Read the model definition and answer for the solid it produces. Units are mm, in the model's axes. Give positions to 0.01 mm unless a question says otherwise; leave off trailing zeros. Loops run counter-clockwise (first coordinate to the right, second up) from the corner with the lowest first, then second, coordinate; pieces in that order, holes last. Notation, with made-up numbers: (74, -12) - (128, -12) arc R19 ccw to (128, 0) - close; hole circle Ø7 at (-33, 36.25). An arc over 180 degrees is marked (long way). Use a Markdown table: item, result. Add a question column.
Item 1: A cutting plane is placed at D-D (z = 2.25). Give the number of separate pieces and of enclosed holes in the cut face, plus the area to 3 significant figures.
Item 2: A cutting plane is placed at A-A (x = 0). Determine the outline of the cut face in (y, z).
Item 3: Each of these flat-tipped pins is pushed along its axis until it touches: P1, Ø1.5, axis at x = 10, z = 2, coming from the -Y side; P2, Ø3, axis at y = -18, z = 1.5, coming from the +X side; P3, Ø2, axis at x = 0.5, z = 3.5, coming from the +Y side. Where does it stop, or does it pass through?
Item 4: Consider probe 1 along Y at (x, z) = (0, 3.2); probe 2 along X at (y, z) = (11.5, 1.15); probe 3 along X at (y, z) = (13, 1.2). Determine where each line is inside the solid, lowest interval first. Write a range as [from, to].
Item 5: A cutting plane is placed at C-C (x = 15). Determine the outline of the cut face in (y, z).
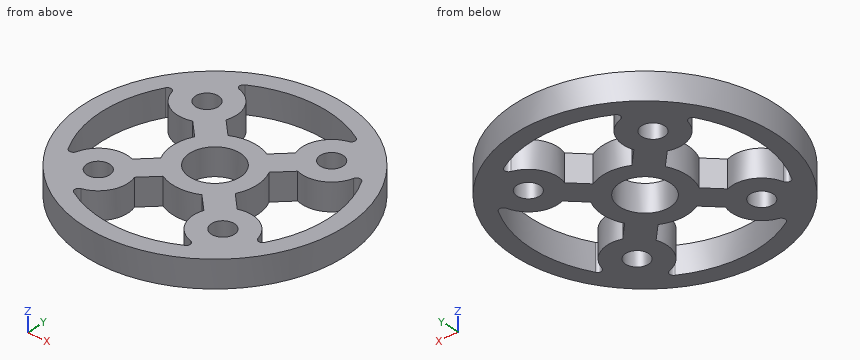
from build123d import *

# Parameters (mm, degrees)
F0_R            = 24.51608
F0_R_2          = 2.15265
F0_R_3          = 4.7625
F1_DEPTH        = 5.08
F3_DEPTH        = 5.08
F3_COPIES_COUNT = 4
F4_R            = 0.762


# Not quite as in the source:
# - a pattern or mirror of a feature is missing from the dataset's text; its kind, count and spacing are read off the source's solid


with BuildPart() as f1:
    # F0 (on Top) → F1 (new body)
    with BuildSketch(Plane.XY):
        Circle(F0_R)
        with Locations((-11.7865906, -11.7865906)):
            Circle(F0_R_2, mode=Mode.SUBTRACT)
        with Locations((11.7865906, -11.7865906)):
            Circle(F0_R_2, mode=Mode.SUBTRACT)
        with Locations((-11.7865906, 11.7865906)):
            Circle(F0_R_2, mode=Mode.SUBTRACT)
        Circle(F0_R_3, mode=Mode.SUBTRACT)
        with Locations((11.7865906, 11.7865906)):
            Circle(F0_R_2, mode=Mode.SUBTRACT)
    extrude(amount=F1_DEPTH)

    # F2 (on face) → F3 (cut, through all)
    with BuildSketch(Plane.XY.offset(5.08)):
        with BuildLine():
            ThreePointArc((-12.5005198818, 17.2967828873), (-7.4612395718, 15.2741760893), (-6.553034663, 9.9206307084))
            Line((-6.553034663, 9.9206307084), (-3.6703384477, 7.0379344931))
            ThreePointArc((-3.6703384477, 7.0379344931), (0, 7.9375), (3.6703384477, 7.0379344931))
            Line((3.6703384477, 7.0379344931), (6.553034663, 9.9206307084))
            ThreePointArc((6.553034663, 9.9206307084), (7.4612395718, 15.2741760893), (12.5005198818, 17.2967828873))
            ThreePointArc((12.5005198818, 17.2967828873), (0, 21.34108), (-12.5005198818, 17.2967828873))
        make_face()
    f3 = extrude(amount=-F3_DEPTH, mode=Mode.SUBTRACT)

    # F3_copies: F3 ×4 about axis
    f3_copies_axis = Axis((0, 0, 0), (0, 0, 1))
    for i in range(1, F3_COPIES_COUNT):
        add(f3.rotate(f3_copies_axis, i * 360 / F3_COPIES_COUNT), mode=Mode.SUBTRACT)

    # F4
    f4_edges = [f1.edges().sort_by_distance(p)[0] for p in [
        (-12.50052, 17.296783, 2.54),
        (12.50052, 17.296783, 2.54),
        (-17.296783, -12.50052, 2.54),
        (-17.296783, 12.50052, 2.54),
        (12.50052, -17.296783, 2.54),
        (-12.50052, -17.296783, 2.54),
        (17.296783, 12.50052, 2.54),
        (17.296783, -12.50052, 2.54),
    ]]
    fillet(f4_edges, radius=F4_R)


solid = f1.part
Geometry says:
| question | item | result |
|---|---|---|
| 1 | separate pieces | 1 |
| 1 | enclosed holes | 9 |
| 1 | area | 971 mm² |
| 2 | outline | (-24.52, 0) - (-21.34, 0) - (-21.34, 5.08) - (-24.52, 5.08) - close; (-7.94, 0) - (-4.76, 0) - (-4.76, 5.08) - (-7.94, 5.08) - close; (4.76, 0) - (7.94, 0) - (7.94, 5.08) - (4.76, 5.08) - close; (21.34, 0) - (24.52, 0) - (24.52, 5.08) - (21.34, 5.08) - close |
| 3 | P1 | y = -22.7 |
| 3 | P2 | x = 18.13 |
| 3 | P3 | y = 24.52 |
| 4 | probe 1 | [-24.52, -21.34], [-7.94, -4.76], [4.76, 7.94], [21.34, 24.52] |
| 4 | probe 2 | [-21.65, -13.92], [-9.65, -6.24], [6.24, 9.65], [13.92, 21.65] |
| 4 | probe 3 | [-20.79, -13.56], [-10.01, -6.36], [6.36, 10.01], [13.56, 20.79] |
| 5 | outline | (-19.39, 0) - (-7.25, 0) - (-7.25, 5.08) - (-19.39, 5.08) - close; (7.25, 0) - (19.39, 0) - (19.39, 5.08) - (7.25, 5.08) - close |
